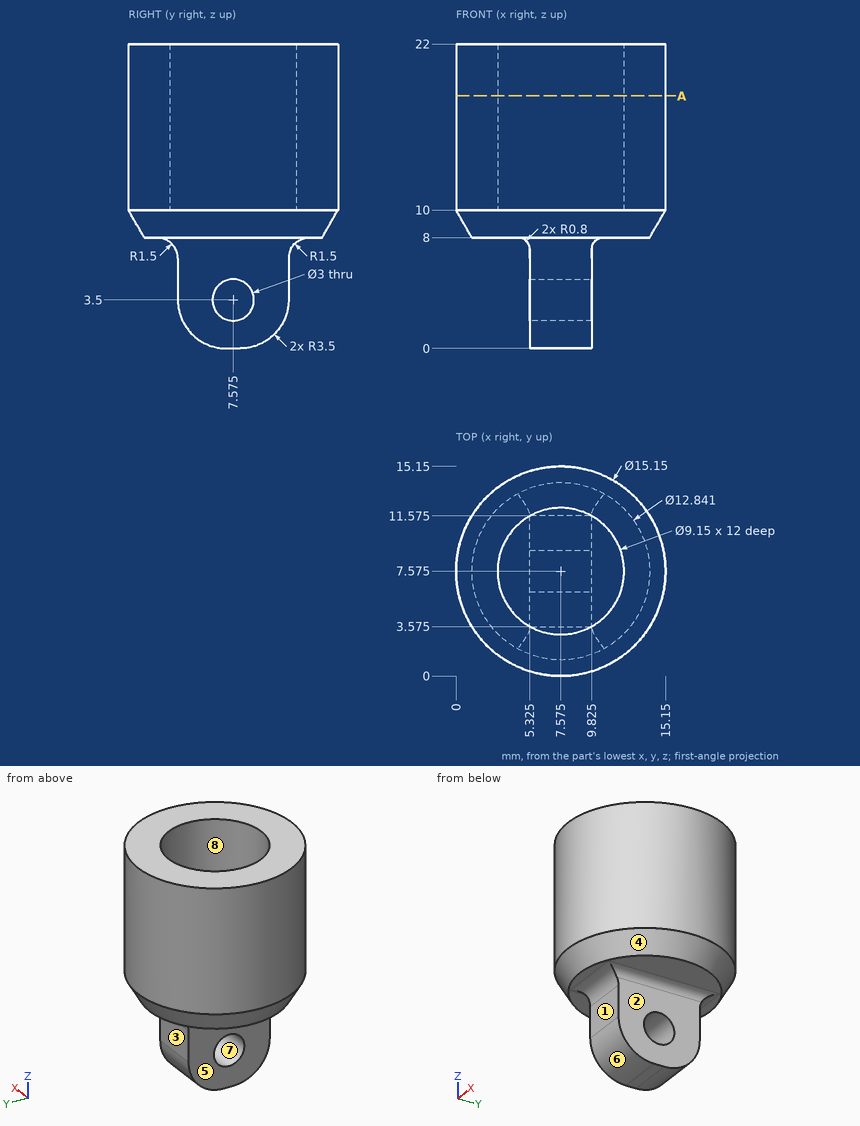
Could you check a few things on this drawing? It's one solid part, dimensions in mm from its lowest x, y, z. A direction names the side the tool comes from. Coordinates: 2 decimals unless noted, no trailing zeros. Loops run counter-clockwise (first coordinate to the right, second up) from the corner with the lowest first, then second, coordinate; pieces in that order, holes last.
1. I need wall thicknesses on L1, parallel to Z at x = 12, y = 11; L2, parallel to X at y = 8, z = 18; L3, parallel to Y at x = 10, z = 20 (1 decimal). Which ranges of each line are inside material? Lowest first, please.
2. We'd pull the mould along Y, two halves only. Please class the marked faces 5, 6, 7 and 8: released by +Y, released by -Y, zero draft, split by the parting line, or undercut.
3. Imagine slicing it at A-A (z = 18.25). Please give me the cut outline in (x, y) (3 decimals), and give its area (4 significant figures).
4. For the marked faces 1, 2, 3 and 4, which set-ups out of +Z, -Z, +X, -X, +Y, -Y let a thin tool reach every point of the face, with its end or its side?
5. For P1, Ø6, axis at y = 7, z = 5.5, coming from the -X side; P2, Ø2.5, axis at x = 8, z = 5.5, coming from the -Y side; P3, Ø8, axis at x = 11, z = 3, coming from the -Y side, each with a flat end and sliding along its axis, tell me the tip position at first contact or that it passes through.
Computed values:
1. L1: z = 8 to 22
1. L2: x = 0.01 to 3.02, 12.13 to 15.14
1. L3: y = 0.4 to 3.7, 11.5 to 14.8
2. face 5: zero draft
2. face 6: released by -Y
2. face 7: undercut
2. face 8: undercut
3. outline: circle Ø15.15 at (7.575, 7.575); hole circle Ø9.15 at (7.575, 7.575)
3. area: 114.5 mm2
4. face 1: -Z, +X, -X, -Y
4. face 2: -Z, +X, +Y, -Y
4. face 3: -Z, +X, -X, +Y
4. face 4: -Z
5. P1: stops at x = 0.88
5. P2: stops at y = 3.55
5. P3: stops at y = 3.54
